Read the model definition and answer for the solid it produces. Units are mm, in the model's axes. Coordinates: 2 decimals unless noted, no trailing zeros. Order: outer loops, then holes, each group sorted by start corner. A loop starts at its lowest first (then second) coordinate and runs counter-clockwise, first axis right, second up. Notation, with made-up numbers: (45, 36.25) - (84, 36.25) arc R22 ccw to (84, 71.25) - close; hole circle Ø5 at (21, 78.25). An arc over 180 degrees is marked (long way). Answer as a JSON object with one key per item and string values. Group by question number.
from build123d import *

# Parameters (mm, degrees)
SKETCH1_W           = 347.4626
SKETCH1_H           = 123.6255
BOSS_EXTRUDE1_DEPTH = 5


with BuildPart() as part:
    # Sketch1 → Boss-Extrude1 (new body)
    with BuildSketch(Plane(origin=(0, 0, 0), x_dir=(1, 0, 0), z_dir=(0, 1, 0))):
        Polygon((382.958, 164.299), (383.35, 164.284), (383.741, 164.237), (384.126, 164.162), (384.503, 164.055), (384.87, 163.919), (385.226, 163.755), (385.572, 163.564), (385.897, 163.344), (386.203, 163.102), (386.493, 162.834), (386.761, 162.547), (387.004, 162.238), (387.223, 161.913), (387.414, 161.569), (387.576, 161.212), (387.713, 160.845), (387.819, 160.467), (387.897, 160.082), (387.943, 159.693), (387.96, 159.299), (387.96, 5.27237), (387.943, 4.881), (387.897, 4.49104), (387.819, 4.10655), (387.713, 3.72759), (387.576, 3.35966), (387.414, 3.00412), (387.223, 2.66099), (387.004, 2.3344), (386.761, 2.02572), (386.493, 1.73771), (386.203, 1.47037), (385.897, 1.22783), (385.572, 1.0101), (385.226, 0.818554), (384.87, 0.654569), (384.503, 0.518142), (384.126, 0.412034), (383.741, 0.334863), (383.35, 0.289388), (382.958, 0.272852), (5.09598, 0.272852), (4.70186, 0.289388), (4.3119, 0.334863), (3.9274, 0.412034), (3.54983, 0.518142), (3.18189, 0.654569), (2.82498, 0.818554), (2.48185, 1.0101), (2.15663, 1.22783), (1.84795, 1.47037), (1.55994, 1.73771), (1.2926, 2.02572), (1.05006, 2.3344), (0.830957, 2.66099), (0.63941, 3.00412), (0.475424, 3.35966), (0.338998, 3.72759), (0.232888, 4.10655), (0.157097, 4.49104), (0.110243, 4.881), (0.0950846, 5.27375), (0.0950846, 159.299), (0.110243, 159.693), (0.157097, 160.082), (0.232888, 160.467), (0.338998, 160.845), (0.475424, 161.212), (0.63941, 161.569), (0.830957, 161.913), (1.05006, 162.238), (1.2926, 162.547), (1.55994, 162.834), (1.84795, 163.102), (2.15663, 163.344), (2.48185, 163.564), (2.82498, 163.755), (3.18189, 163.919), (3.54983, 164.055), (3.9274, 164.162), (4.3119, 164.237), (4.70186, 164.284), (5.09598, 164.299), align=None)
        with Locations((194.0257, 82.28625)):
            Rectangle(SKETCH1_W, SKETCH1_H, mode=Mode.SUBTRACT)
    extrude(amount=BOSS_EXTRUDE1_DEPTH)


solid = part.part
1. A cutting plane is placed at B-B on z = -78.5. Write down the section's boundary in (x, y), and give its area (3 significant figures).
2. Given pin 1 (8 mm diameter, centred on x = 51.5, z = -140, fed in from -Y), flat-ended and moving along its own axis, determine where the tip first touches the part or whether it passes through.
3. Straight lines are drawn through the part: L1, parallel to Z at x = 124, y = 1.85; L2, parallel to X at y = 1.65, z = -143.5. For each, find the intervals that lie inside material, in ascending order.
4. A cutting plane is placed at A-A on x = 278.5. Write down the section's boundary in (y, z), and give its area (3 significant figures).
Derived:
{
 "1": {"outline": "(0.1, 0) - (20.29, 0) - (20.29, 5) - (0.1, 5) - close; (367.76, 0) - (387.96, 0) - (387.96, 5) - (367.76, 5) - close", "area": "202 mm2"},
 "2": {"pin 1": "passes through"},
 "3": {"L1": "z = -164.3 to -144.1, -20.47 to -0.27", "L2": "x = 0.1 to 20.29, 367.76 to 387.96"},
 "4": {"outline": "(0, -164.3) - (5, -164.3) - (5, -144.1) - (0, -144.1) - close; (0, -20.47) - (5, -20.47) - (5, -0.27) - (0, -0.27) - close", "area": "202 mm2"}
}
